Drawing for the job (mm, zero at the part's lowest x, y, z). A direction names the side the tool comes from. Give positions to 0.01 mm unless a question says otherwise; leave off trailing zeros. Loops run counter-clockwise (first coordinate to the right, second up) from the corner with the lowest first, then second, coordinate; pieces in that order, holes last. Notation, with made-up numbers: (-36.5, 50.25) -> (7.5, 50.25) arc R11 cw to (7.5, 58.25) -> close; hole circle Ø4 at (59.5, 51). An arc over 180 degrees is marked (long way). Write item = value, one per line.
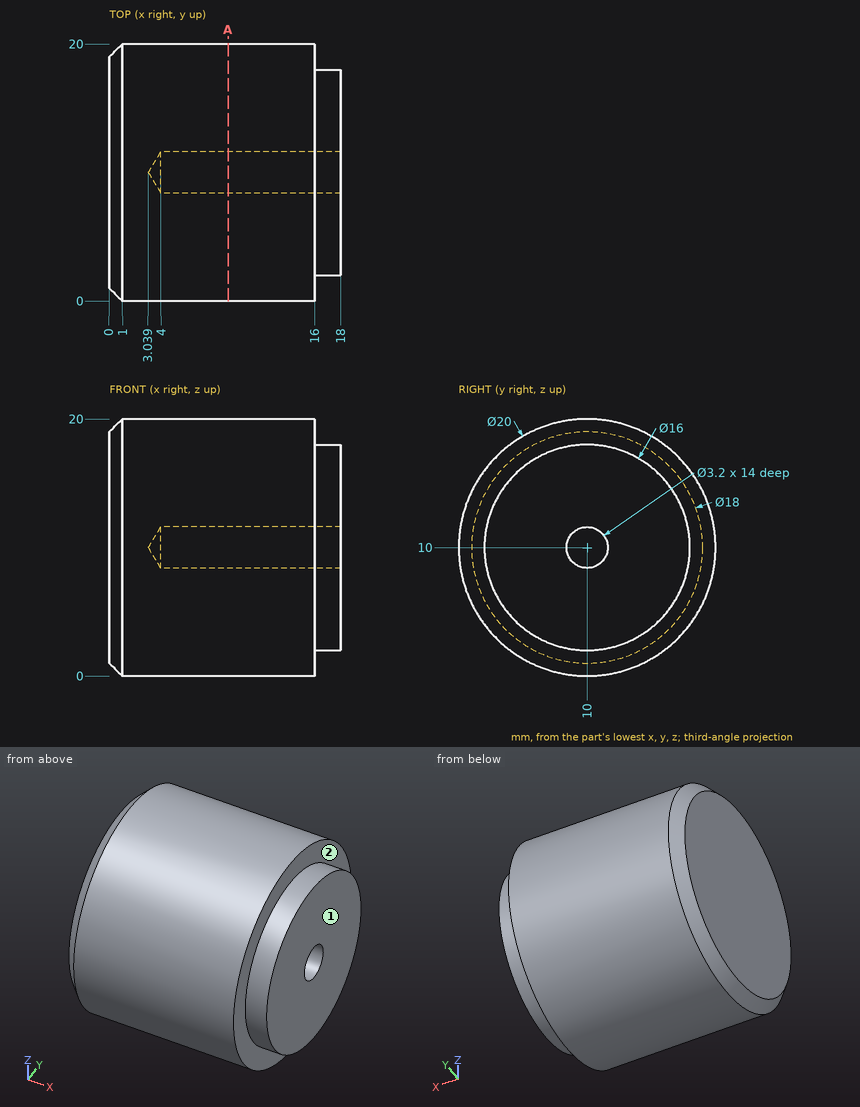
1) Drill centre lines: line 1 along Z through (x, y) = (9.5, 10); line 2 along Z through (x, y) = (5.75, 18); line 3 along X through (y, z) = (2.75, 14). Where is each one in solid material? Low to high. Write a range as [from, to].
Resolved:
line_1 = [0, 8.4], [11.6, 20]
line_2 = [4, 16]
line_3 = [0, 16]
2) Slice it at A-A, the plane x = 9.25. List the corners of the cut face in (y, z).
Resolved:
outline = circle Ø20 at (10, 10); hole circle Ø3.2 at (10, 10)
3) Drop flat-ended pins along their axis: P1, Ø4, axis at x = 10.5, z = 15, coming from the -Y side; P2, Ø1, axis at x = 5, z = 2.5, coming from the -Y side; P3, Ø4, axis at x = 14, z = 15.5, coming from the -Y side. Give the stop position or say it passes through.
Resolved:
P1 = 0.46
P2 = 2.86
P3 = 0.63
4) Which spindle directions (+Z, -Z, +X, -X, +Y, -Y) get a long thin tool onto all of the face, cutting with end or side? Do the marked faces 1 and 2. Say none if no direction does.
Resolved:
face_1 = +Z, -Z, +X, +Y, -Y
face_2 = +X
